```python
from build123d import *

# Parameters (mm, degrees)
F0_W     = 65
F0_H     = 30
F1_DEPTH = 150
F2_R     = 10
F3_T     = -1.5
F4_DEPTH = 1.5
F5_W     = 6
F5_H     = 6
F6_DEPTH = 65.001


with BuildPart() as f1:
    # F0 (on Top) → F1 (new body)
    with BuildSketch(Plane.XY):
        with Locations((32.5, -15)):
            Rectangle(F0_W, F0_H)
    extrude(amount=F1_DEPTH)

    # F2
    f2_edges = [f1.edges().sort_by_distance(p)[0] for p in [
        (65, 0, 75),
        (65, -30, 75),
        (0, 0, 75),
        (0, -30, 75),
    ]]
    fillet(f2_edges, radius=F2_R)

    # F3
    f3_openings = [f1.faces().sort_by_distance(p)[0] for p in [
        (32.5, -15, 150),
    ]]
    offset(amount=F3_T, openings=f3_openings)

    # F4 (cut, through all): a face of the model
    f4_faces = [f1.faces().sort_by_distance(p)[0] for p in [
        (32.5, -15, 1.5),
    ]]
    extrude(f4_faces, amount=-F4_DEPTH, mode=Mode.SUBTRACT)

    # F5 (on face) → F6 (cut, through all)
    with BuildSketch(Plane(origin=(0, 0, 0), x_dir=(0, -1, 0), z_dir=(-1, 0, 0))):
        with Locations((15, 18)):
            Rectangle(F5_W, F5_H)
        with Locations((15, 132)):
            Rectangle(F5_W, F5_H)
    extrude(amount=-F6_DEPTH, mode=Mode.SUBTRACT)


solid = f1.part
```
Geometry: final body of the model. Coordinates: model frame, mm. A direction names the side the tool comes from. Coordinates: 2 decimals unless noted, no trailing zeros. Order: outer loops, then holes, each group sorted by start corner. A loop starts at its lowest first (then second) coordinate and runs counter-clockwise, first axis right, second up. Notation, with made-up numbers: (76, 0.25) - (80, 0.25) arc R27 ccw to (80, 33.25) - close; hole circle Ø6 at (77.5, 78.25). An arc over 180 degrees is marked (long way). Return JSON: item names as keys, results as strings. Group by question number.
1. Pull-direction query (X, two-part tool) for faces 3 (the face through (0, -15, 74)), 4 (the face through (62.15, -3.01, 76.05)), 5 (the face through (3.92, -25.94, 76.05)); classes: pulls with the +X half, pulls with the -X half, needs draft (parallel to the pull), parting line crosses it, or undercut.
2. Material intervals for line 1 along Y through (x, z) = (50, 84); line 2 along X through (y, z) = (-15, 38.5); line 3 along X through (y, z) = (-26.5, 40), sorted ascending. Write a range as [from, to].
3. Set-up query: faces 1 (the face through (2.85, -3.01, 76.05)), 2 (the face through (63.5, -15, 76)). Return all of +Z, -Z, +X, -X, +Y, -Y with unobstructed straight access to the full face (end or side cutting, diameter ignored); none if empty.
4. Cut plane C-C (z = 64). Output: boundary loops of the cut face in (x, y).
5. Cut plane A-A (y = -16). Output: boundary loops of the cut face in (x, z).
6. Cut plane B-B (x = 50). Output: boundary loops of the cut face in (y, z), plus the area to 3 significant figures.
7. Cut plane D-D (y = -23.5). Output: boundary loops of the cut face in (x, z), plus the area to 3 significant figures.
8. Pin query (flat end, axial travel): pin 1 (4 mm diameter, centred on y = -25.5, z = 46.5, fed in from -X); pin 2 (0.8 mm diameter, centred on x = 0.5, z = 132.5, fed in from +Y); pin 3 (0.8 mm diameter, centred on x = 64.5, y = -16, fed in from -Z); pin 4 (1.2 mm diameter, centred on x = 0.5, z = 133, fed in from -Y). Return the tip coordinate at first contact, or that it passes through.
Resolved:
{
 "1": {"face 3": "pulls with the -X half", "face 4": "pulls with the +X half", "face 5": "undercut"},
 "2": {"line 1": "y = [-30, -28.5], [-1.5, 0]", "line 2": "x = [0, 1.5], [63.5, 65]", "line 3": "x = [2.4, 4.52], [60.48, 62.6]"},
 "3": {"face 1": "+Z, -Z, -X, +Y", "face 2": "+Z, -Z"},
 "4": {"outline": "(0, -20) arc R10 ccw to (10, -30) - (55, -30) arc R10 ccw to (65, -20) - (65, -10) arc R10 ccw to (55, 0) - (10, 0) arc R10 ccw to (0, -10) - close; hole (1.5, -20) arc R8.5 ccw to (10, -28.5) - (55, -28.5) arc R8.5 ccw to (63.5, -20) - (63.5, -10) arc R8.5 ccw to (55, -1.5) - (10, -1.5) arc R8.5 ccw to (1.5, -10) - close"},
 "5": {"outline": "(0, 0) - (1.5, 0) - (1.5, 15) - (0, 15) - close; (0, 21) - (1.5, 21) - (1.5, 129) - (0, 129) - close; (0, 135) - (1.5, 135) - (1.5, 150) - (0, 150) - close; (63.5, 0) - (65, 0) - (65, 15) - (63.5, 15) - close; (63.5, 21) - (65, 21) - (65, 129) - (63.5, 129) - close; (63.5, 135) - (65, 135) - (65, 150) - (63.5, 150) - close"},
 "6": {"outline": "(-30, 0) - (-28.5, 0) - (-28.5, 150) - (-30, 150) - close; (-1.5, 0) - (0, 0) - (0, 150) - (-1.5, 150) - close", "area": "450 mm²"},
 "7": {"outline": "(0.63, 0) - (2.25, 0) - (2.25, 150) - (0.63, 150) - close; (62.75, 0) - (64.37, 0) - (64.37, 150) - (62.75, 150) - close", "area": "486 mm²"},
 "8": {"pin 1": "stops at x = 0.63", "pin 2": "stops at y = -5.85", "pin 3": "stops at z = 0", "pin 4": "stops at y = -24.56"}
}
